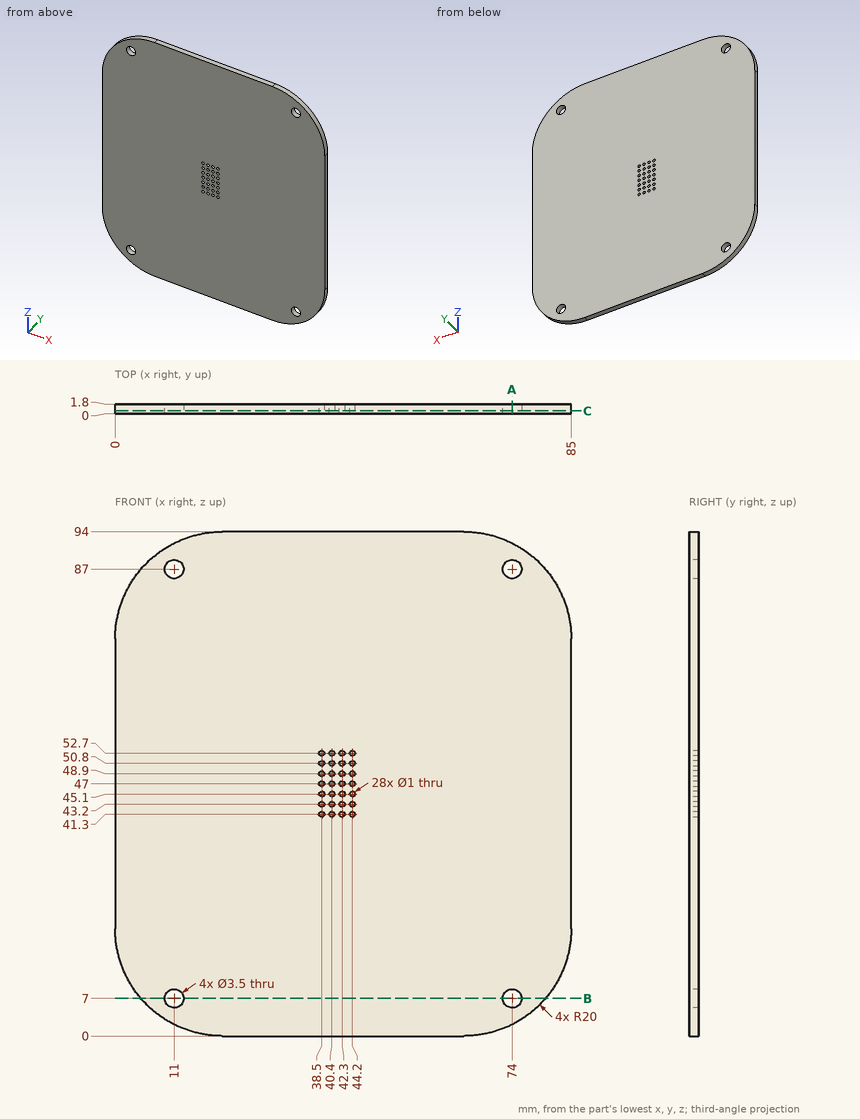
The figure shows three views and two pictorial views of one solid part (mm, origin at its lowest corner). Answer the questions. Round coordinates to 2 decimals unless told otherwise and drop trailing zeros. Loops run counter-clockwise (first coordinate to the right, second up) from the corner with the lowest first, then second, coordinate; pieces in that order, holes last. Notation, with made-up numbers: M 87.5,80 L 132.5,80 A29 cw 132.5,105 Z; hole C 67,23 d7. An arc over 180 degrees is marked long. Return JSON: item names as keys, results as strings.
Q1. Find the intervals of material crossed by line 1 along X through (y, z) = (1.25, 52.7); line 2 along Z through (x, y) = (11, 0.75); line 3 along Z through (x, y) = (75, 1.4), in increasing order. Write a range as from..to.
Results list:
{"line 1": "x = 0..38, 39..39.9, 40.9..41.8, 42.8..43.7, 44.7..85", "line 2": "z = 2.14..5.25, 8.75..85.25, 88.75..91.86", "line 3": "z = 2.68..5.56, 8.44..85.56, 88.44..91.32"}
Q2. Find section C-C, the plane y = 0.5. State how many separate pieces and enclosed holes the cut face has, plus the area to 3 significant figures.
Results list:
{"separate pieces": "1", "enclosed holes": "32", "area": "7,590 mm2"}
Q3. Find section B-B, the plane z = 7. Determine the outline of the cut face in (x, y), plus the area to 3 significant figures.
Results list:
{"outline": "M 4.8,0 L 9.25,0 L 9.25,1.8 L 4.8,1.8 Z; M 12.75,0 L 72.25,0 L 72.25,1.8 L 12.75,1.8 Z; M 75.75,0 L 80.2,0 L 80.2,1.8 L 75.75,1.8 Z", "area": "123 mm2"}
Q4. Find section A-A, the plane x = 74. Determine the outline of the cut face in (y, z).
Results list:
{"outline": "M 0,2.14 L 1.8,2.14 L 1.8,5.25 L 0,5.25 Z; M 0,8.75 L 1.8,8.75 L 1.8,85.25 L 0,85.25 Z; M 0,88.75 L 1.8,88.75 L 1.8,91.86 L 0,91.86 Z"}
Q5. Each of these flat-tipped pins is pushed along its axis until it touches: pin 1 Ø4 at (x, z) = (74, 87) entering from +Y; pin 2 Ø1 at (y, z) = (0.5, 18.5) entering from +X (3 decimals). Where does it stop, or does it pass through?
Results list:
{"pin 1": "stops at y = 1.8", "pin 2": "stops at x = 84.975"}
